Geometry check sheet. Reference: the model listing, model coordinates, mm. A direction names the side the tool comes from. Round coordinates to 2 decimals unless told otherwise and drop trailing zeros. Loops run counter-clockwise (first coordinate to the right, second up) from the corner with the lowest first, then second, coordinate; pieces in that order, holes last. Notation, with made-up numbers: (59.25, 4) -> (101.25, 4) arc R11 cw to (101.25, 17) -> close; hole circle Ø10 at (3.5, 75). An arc over 180 degrees is marked (long way). Use one line per item in the form item = value.
from build123d import *

# Parameters (mm, degrees)
F0_W     = 218.84298
F0_H     = 170.608
F1_DEPTH = 5
F2_D     = 4
F3_W     = 70
F3_H     = 8
F4_DEPTH = 50


with BuildPart() as f1:
    # F0 (on Top) → F1 (new body)
    with BuildSketch(Plane.XY):
        with Locations((4.32045, 0.03)):
            Rectangle(F0_W, F0_H)
    extrude(amount=F1_DEPTH)

    # F2 (through all)
    with Locations(Plane(origin=(0, 0, 0), x_dir=(1, 0, 0), z_dir=(0, 0, -1))):
        with Locations((-75.883113, 42.666), (0, 77.334), (89.466453, 42.666), (-75.883113, -42.666), (0, -77.334), (89.466453, -42.666)):
            Hole(F2_D / 2)

    # F3 (on Right) → F4 (join, symmetric)
    with BuildSketch(Plane.YZ):
        with Locations((0, -4)):
            Rectangle(F3_W, F3_H)
    extrude(amount=F4_DEPTH, both=True)


solid = f1.part
1. Material ranges on line 1 along X through (y, z) = (42.5, 0.25); line 2 along Y through (x, z) = (0, 3.05); line 3 along Z through (x, y) = (-51, 44), recorded low to high.
Return value:
line_1 = -105.1 to -77.88, -73.89 to 87.47, 91.46 to 113.74
line_2 = -85.27 to -79.33, -75.33 to 75.33, 79.33 to 85.33
line_3 = 0 to 5
2. Section check D-D (y = 37.5). Record the boundary of the cut face in (x, z).
Return value:
outline = (-105.1, 0) -> (113.74, 0) -> (113.74, 5) -> (-105.1, 5) -> close
3. Section check C-C (z = -2.25). Record the boundary of the cut face in (x, y), then the cut area to 3 significant figures.
Return value:
outline = (-50, -35) -> (50, -35) -> (50, 35) -> (-50, 35) -> close
area = 7,000 mm2
4. Tool access check on faces 1 (the flat face through (50, 0, -4)), 2 (the flat face through (-50, 0, -4)), 3 (the flat face through (1, 35, -4)). Record the directions out of +Z, -Z, +X, -X, +Y, -Y that give a thin tool (end or side, any length) a straight path to the whole face; none if there is none.
Return value:
face_1 = -Z, +X, +Y, -Y
face_2 = -Z, -X, +Y, -Y
face_3 = -Z, +X, -X, +Y
5. Section check B-B (x = 39). Record the boundary of the cut face in (y, z).
Return value:
outline = (-85.27, 0) -> (-35, 0) -> (-35, -8) -> (35, -8) -> (35, 0) -> (85.33, 0) -> (85.33, 5) -> (-85.27, 5) -> close
6. Gauge pin test, flat ends, axial feed: pin 1 (4 mm diameter, centred on y = -7, z = -3, fed in from +X); pin 2 (5 mm diameter, centred on x = -75.88, y = -42.67, fed in from -Z); pin 3 (2 mm diameter, centred on x = -34, z = -2, fed in from -Y); pin 4 (3.5 mm diameter, centred on x = 89.47, y = -42.67, fed in from -Z). Record the tip position at first contact, or that the pin passes through.
Return value:
pin_1 = 50
pin_2 = 0
pin_3 = -35
pin_4 = through
7. Section check A-A (y = 0). Record the boundary of the cut face in (x, z).
Return value:
outline = (-105.1, 0) -> (-50, 0) -> (-50, -8) -> (50, -8) -> (50, 0) -> (113.74, 0) -> (113.74, 5) -> (-105.1, 5) -> close
